Read the model definition and answer for the solid it produces. Units are mm, in the model's axes. Face numbers are marked on the shaded views. A direction names the side the tool comes from. Coordinates: 2 decimals unless noted, no trailing zeros. Answer as a JSON object with one key per item and string values. Group by question number.
1) Determine the mould class of the marked faces 3 and 4 for opening direction Y: released by +Y, released by -Y, zero draft, split by the parting line, or undercut.
2) Section A-A on y = -257 is taken. Count the separate pieces of the cut face and the enclosed holes in it, and give its area (3 significant figures).
3) A tool of negligible diameter and unlimited length cuts with its end or side. For the marked faces 1 and 2, from which of +Z, -Z, +X, -X, +Y, -Y can it reach the whole face along a straight path? Write none if from no direction.
4) Given pin 1 (1.5 mm diameter, centred on x = 396, z = 2, fed in from -Y); pin 2 (1 mm diameter, centred on x = 388, z = 2, fed in from +Y); pin 3 (1.5 mm diameter, centred on x = 396, z = 1, fed in from +Y), each flat-ended and moving along its own axis, determine where each tip first touches the part or whether it passes through.
5) Consider L1, parallel to X at y = -270, z = 0.65; L2, parallel to Y at x = 403.25, z = 1.1; L3, parallel to X at y = -264.5, z = 1. Determine where each line is inside the solid, lowest interval first.
from build123d import *

# Parameters (mm, degrees)
SALIENTE_EXTRUIR1_DEPTH = 3


with BuildPart() as part:
    # Croquis1 → Saliente-Extruir1 (new body)
    with BuildSketch(Plane.XY):
        with BuildLine():
            add(Edge.make_bspline(
                [(389.936156465, -257.964269658), (389.256388965, -256.299793547), (387.405469799, -255.444131047), (385.697178688, -256.004589103)],
                knots=[0, 0, 0, 0, 1, 1, 1, 1], degree=3))
            add(Edge.make_bspline(
                [(385.697178688, -256.004589103), (385.614134799, -256.11479688), (385.533031188, -256.226451047), (385.453832577, -256.339481047)],
                knots=[0, 0, 0, 0, 1, 1, 1, 1], degree=3))
            add(Edge.make_bspline(
                [(385.453832577, -256.339481047), (385.448752577, -258.137377713), (386.834498966, -259.633261324), (388.627527299, -259.76541188)],
                knots=[0, 0, 0, 0, 1, 1, 1, 1], degree=3))
            add(Edge.make_bspline(
                [(388.627527299, -259.76541188), (388.245751188, -260.49993049), (387.988188132, -261.292586879), (387.86535091, -262.111207712)],
                knots=[0, 0, 0, 0, 1, 1, 1, 1], degree=3))
            add(Edge.make_bspline(
                [(387.86535091, -262.111207712), (386.337047021, -261.164211046), (384.336691189, -261.559886601), (383.284037578, -263.017423268)],
                knots=[0, 0, 0, 0, 1, 1, 1, 1], degree=3))
            add(Edge.make_bspline(
                [(383.284037578, -263.017423268), (383.281673967, -263.155394656), (383.281673967, -263.293401323), (383.284037578, -263.431372712)],
                knots=[0, 0, 0, 0, 1, 1, 1, 1], degree=3))
            add(Edge.make_bspline(
                [(383.284037578, -263.431372712), (384.336691189, -264.888909378), (386.337047021, -265.284584934), (387.86535091, -264.337588267)],
                knots=[0, 0, 0, 0, 1, 1, 1, 1], degree=3))
            add(Edge.make_bspline(
                [(387.86535091, -264.337588267), (387.988188132, -265.1562091), (388.245751188, -265.948865489), (388.627527299, -266.6833841)],
                knots=[0, 0, 0, 0, 1, 1, 1, 1], degree=3))
            add(Edge.make_bspline(
                [(388.627527299, -266.6833841), (386.834498966, -266.815534656), (385.448752577, -268.311418266), (385.453832577, -270.109314932)],
                knots=[0, 0, 0, 0, 1, 1, 1, 1], degree=3))
            add(Edge.make_bspline(
                [(385.453832577, -270.109314932), (385.533031188, -270.222344932), (385.614134799, -270.333999099), (385.697178688, -270.444206877)],
                knots=[0, 0, 0, 0, 1, 1, 1, 1], degree=3))
            add(Edge.make_bspline(
                [(385.697178688, -270.444206877), (387.405469799, -271.004664932), (389.256388965, -270.149002432), (389.936156465, -268.4845616)],
                knots=[0, 0, 0, 0, 1, 1, 1, 1], degree=3))
            add(Edge.make_bspline(
                [(389.936156465, -268.4845616), (390.516722854, -269.074617711), (391.191022298, -269.564484933), (391.931608687, -269.934337155)],
                knots=[0, 0, 0, 0, 1, 1, 1, 1], degree=3))
            add(Edge.make_bspline(
                [(391.931608687, -269.934337155), (390.558668132, -271.095152432), (390.316874243, -273.119885209), (391.377747576, -274.571424654)],
                knots=[0, 0, 0, 0, 1, 1, 1, 1], degree=3))
            add(Edge.make_bspline(
                [(391.377747576, -274.571424654), (391.508240076, -274.616333265), (391.639508687, -274.65894882), (391.771447576, -274.699341876)],
                knots=[0, 0, 0, 0, 1, 1, 1, 1], degree=3))
            add(Edge.make_bspline(
                [(391.771447576, -274.699341876), (393.482948964, -274.148620487), (394.477394242, -272.368433265), (394.049016186, -270.622324377)],
                knots=[0, 0, 0, 0, 1, 1, 1, 1], degree=3))
            add(Edge.make_bspline(
                [(394.049016186, -270.622324377), (394.86555563, -270.758426043), (395.69899313, -270.758426043), (396.515532574, -270.622324377)],
                knots=[0, 0, 0, 0, 1, 1, 1, 1], degree=3))
            add(Edge.make_bspline(
                [(396.515532574, -270.622324377), (396.087119241, -272.368433265), (397.081599797, -274.148620487), (398.793065907, -274.699341876)],
                knots=[0, 0, 0, 0, 1, 1, 1, 1], degree=3))
            add(Edge.make_bspline(
                [(398.793065907, -274.699341876), (398.925040074, -274.65894882), (399.056273407, -274.616333265), (399.186765907, -274.571424654)],
                knots=[0, 0, 0, 0, 1, 1, 1, 1], degree=3))
            add(Edge.make_bspline(
                [(399.186765907, -274.571424654), (400.247674518, -273.119885209), (400.005845351, -271.095152432), (398.632904796, -269.934337155)],
                knots=[0, 0, 0, 0, 1, 1, 1, 1], degree=3))
            add(Edge.make_bspline(
                [(398.632904796, -269.934337155), (399.373526463, -269.564484933), (400.047790629, -269.074617711), (400.628357018, -268.4845616)],
                knots=[0, 0, 0, 0, 1, 1, 1, 1], degree=3))
            add(Edge.make_bspline(
                [(400.628357018, -268.4845616), (401.308124518, -270.149002432), (403.159043684, -271.004664932), (404.867370072, -270.444206877)],
                knots=[0, 0, 0, 0, 1, 1, 1, 1], degree=3))
            add(Edge.make_bspline(
                [(404.867370072, -270.444206877), (404.950378683, -270.333999099), (405.031517572, -270.222344932), (405.110680906, -270.109314932)],
                knots=[0, 0, 0, 0, 1, 1, 1, 1], degree=3))
            add(Edge.make_bspline(
                [(405.110680906, -270.109314932), (405.115796183, -268.311418266), (403.730049795, -266.815534656), (401.936986184, -266.6833841)],
                knots=[0, 0, 0, 0, 1, 1, 1, 1], degree=3))
            add(Edge.make_bspline(
                [(401.936986184, -266.6833841), (402.318762295, -265.948865489), (402.576325351, -265.1562091), (402.699197851, -264.337588267)],
                knots=[0, 0, 0, 0, 1, 1, 1, 1], degree=3))
            add(Edge.make_bspline(
                [(402.699197851, -264.337588267), (404.227466461, -265.284584934), (406.227822294, -264.888909378), (407.280475905, -263.431372712)],
                knots=[0, 0, 0, 0, 1, 1, 1, 1], degree=3))
            add(Edge.make_bspline(
                [(407.280475905, -263.431372712), (407.282874794, -263.293401323), (407.282874794, -263.155394656), (407.280475905, -263.017423268)],
                knots=[0, 0, 0, 0, 1, 1, 1, 1], degree=3))
            add(Edge.make_bspline(
                [(407.280475905, -263.017423268), (406.227822294, -261.559886601), (404.227466461, -261.164211046), (402.699197851, -262.111207712)],
                knots=[0, 0, 0, 0, 1, 1, 1, 1], degree=3))
            add(Edge.make_bspline(
                [(402.699197851, -262.111207712), (402.576325351, -261.292586879), (402.318762295, -260.49993049), (401.936986184, -259.76541188)],
                knots=[0, 0, 0, 0, 1, 1, 1, 1], degree=3))
            add(Edge.make_bspline(
                [(401.936986184, -259.76541188), (403.730049795, -259.633261324), (405.115796183, -258.137377713), (405.110680906, -256.339481047)],
                knots=[0, 0, 0, 0, 1, 1, 1, 1], degree=3))
            add(Edge.make_bspline(
                [(405.110680906, -256.339481047), (405.031517572, -256.226451047), (404.950378683, -256.11479688), (404.867370072, -256.004589103)],
                knots=[0, 0, 0, 0, 1, 1, 1, 1], degree=3))
            add(Edge.make_bspline(
                [(404.867370072, -256.004589103), (403.159043684, -255.444131047), (401.308124518, -256.299793547), (400.628357018, -257.964269658)],
                knots=[0, 0, 0, 0, 1, 1, 1, 1], degree=3))
            add(Edge.make_bspline(
                [(400.628357018, -257.964269658), (400.047790629, -257.374178269), (399.373526463, -256.884311047), (398.632904796, -256.514458825)],
                knots=[0, 0, 0, 0, 1, 1, 1, 1], degree=3))
            add(Edge.make_bspline(
                [(398.632904796, -256.514458825), (400.005845351, -255.353643547), (400.247674518, -253.32891077), (399.186765907, -251.877371326)],
                knots=[0, 0, 0, 0, 1, 1, 1, 1], degree=3))
            add(Edge.make_bspline(
                [(399.186765907, -251.877371326), (399.056273407, -251.832462715), (398.925040074, -251.789847159), (398.793065907, -251.749454104)],
                knots=[0, 0, 0, 0, 1, 1, 1, 1], degree=3))
            add(Edge.make_bspline(
                [(398.793065907, -251.749454104), (397.081599797, -252.300175492), (396.087119241, -254.080362714), (396.515532574, -255.826471603)],
                knots=[0, 0, 0, 0, 1, 1, 1, 1], degree=3))
            add(Edge.make_bspline(
                [(396.515532574, -255.826471603), (395.69899313, -255.690369936), (394.86555563, -255.690369936), (394.049016186, -255.826471603)],
                knots=[0, 0, 0, 0, 1, 1, 1, 1], degree=3))
            add(Edge.make_bspline(
                [(394.049016186, -255.826471603), (394.477394242, -254.080362714), (393.482948964, -252.300175492), (391.771447576, -251.749454104)],
                knots=[0, 0, 0, 0, 1, 1, 1, 1], degree=3))
            add(Edge.make_bspline(
                [(391.771447576, -251.749454104), (391.639508687, -251.789847159), (391.508240076, -251.832462715), (391.377747576, -251.877371326)],
                knots=[0, 0, 0, 0, 1, 1, 1, 1], degree=3))
            add(Edge.make_bspline(
                [(391.377747576, -251.877371326), (390.316874243, -253.32891077), (390.558668132, -255.353643547), (391.931608687, -256.514458825)],
                knots=[0, 0, 0, 0, 1, 1, 1, 1], degree=3))
            add(Edge.make_bspline(
                [(391.931608687, -256.514458825), (391.191022298, -256.884311047), (390.516722854, -257.374178269), (389.936156465, -257.964269658)],
                knots=[0, 0, 0, 0, 1, 1, 1, 1], degree=3))
        make_face()
        with BuildLine():
            Line((393.032275353, -264.974387434), (397.532273408, -264.974387434))
            add(Edge.make_bspline(
                [(397.532273408, -264.974387434), (398.332832018, -263.945087712), (398.332832018, -262.503708268), (397.532273408, -261.474408546)],
                knots=[0, 0, 0, 0, 1, 1, 1, 1], degree=3))
            Line((397.532273408, -261.474408546), (393.032275353, -261.474408546))
            add(Edge.make_bspline(
                [(393.032275353, -261.474408546), (392.231681464, -262.503708268), (392.231681464, -263.945087712), (393.032275353, -264.974387434)],
                knots=[0, 0, 0, 0, 1, 1, 1, 1], degree=3))
        make_face(mode=Mode.SUBTRACT)
    extrude(amount=SALIENTE_EXTRUIR1_DEPTH)


solid = part.part
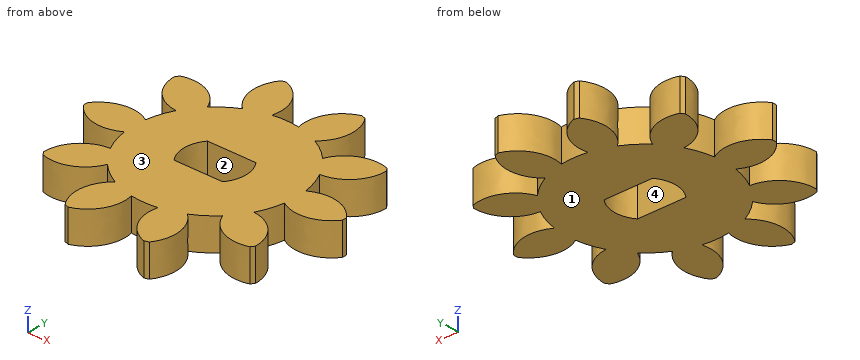
Worked answers:
{
 "1": {"face 3": "zero draft", "face 4": "undercut"},
 "2": {"separate pieces": "3", "enclosed holes": "0", "area": "48.1 mm²"},
 "3": {"face 1": "-Z, +X, -X, +Y, -Y", "face 2": "+Z, -Z"},
 "4": {"pin 1": "stops at y = -272.91", "pin 2": "stops at y = -255.91", "pin 3": "stops at y = -253.54"},
 "5": {"L1": "x = 385.46 to 388.72, 391.86 to 398.71, 401.84 to 405.11", "L2": "y = -270.57 to -267.05, -264.61 to -261.83, -259.4 to -255.88", "L3": "x = 384.55 to 387.57, 387.89 to 392.73, 397.83 to 402.67, 402.99 to 406.02"}
}
